Autodesk Inventor part; units mm, degrees
ref_plane "YZ Plane" through (0, 0, 0) normal (1, 0, 0) x (0, 1, 0)
ref_plane "XZ Plane" through (0, 0, 0) normal (0, 1, 0) x (-1, 0, 0)
ref_plane "XY Plane" through (0, 0, 0) normal (0, 0, 1) x (1, 0, 0)
sketch "Sketch1" plane through (0, 0, 0) normal (1, 0, 0) x (0, 1, 0)
  line L0 (-20, -30) -> (20, -30)
  line L1 (20, -30) -> (20, 30)
  line L2 (20, 30) -> (-20, 30)
  line L3 (-20, 30) -> (-20, -30)
  line L4 (-20, -30) -> (20, 30) construction
  line L5 (20, -30) -> (-20, 30) construction
  circle A0 centre (0, -30) radius 20
  point P0 (0, 0)
  dimension "d0" = 40
  dimension "d1" = 60
extrude "Extrusion1" add sketch "Sketch1" along normal blind 4
sketch "Sketch4" plane through (4, 0, 0) normal (1, 0, 0) x (0, 0, -1)
  line L0 (-5, 20) -> (-90, 20)
  line L1 (-90, 20) -> (-90, -50)
  line L2 (-90, -50) -> (-5, -50)
  line L3 (-5, -50) -> (-5, 20)
  line L4 (0, -64) -> (0, 34)
  line L5 (-10, -77.5279) -> (-10, 43.8166)
  dimension "d40" = 85
  dimension "d41" = 70
  dimension "d54" = 10
  dimension "d55" = 5
extrude "Extrusion4" add sketch "Sketch4" against normal blind 4
sketch "Sketch5" plane through (0, 0, 0) normal (-1, 0, 0) x (0, 0, 1)
  line L0 (34.5, -27) -> (24.2, -27)
  line L1 (24.2, -27) -> (24.2, -22.7)
  line L2 (24.2, -22.7) -> (34.5, -22.7)
  line L3 (34.5, -22.7) -> (34.5, -27)
  line L4 (90, -50) -> (90, -6.689)
  line L5 (90, -50) -> (90, 20)
  line L6 (90, -50) -> (10.2215, -50)
  line L7 (5, -50) -> (90, -50)
  dimension "d20" = 10.3
  dimension "d21" = 4.3
extrude "Extrusion5" cut sketch "Sketch5" against normal blind 4
sketch "Sketch2" plane through (0, 0, 0) normal (-1, 0, 0) x (0, 0, 1)
  arc A0 (-30, 20) -> (-30, -20) centre (-30, 0) ccw
  circle A1 centre (-30, 0) radius 5.15
  point P0 (0, 0)
  dimension "d4" = 10.3
extrude "Extrusion2" cut sketch "Sketch2" against normal blind 4
sketch "Sketch7" plane through (0, 0, 0) normal (-1, 0, 0) x (0, 0, 1)
  circle A0 centre (65, -7.5) radius 22.5
  line L0 (90, -50) -> (90, 20)
  line L1 (-30, 20) -> (90, 20)
  point P0 (0, 0)
  dimension "d47" = 45
  dimension "d48" = 25
  dimension "d53" = 27.5
extrude "Extrusion7" cut sketch "Sketch7" against normal blind 4
fillet "Fillet3" radius 15 2 edges at (2, -20, 5) (2, -50, 5)
properties part number "houder"
Read the model definition and answer for the solid it produces. Units are mm, in the model's axes. A direction names the side the tool comes from. Give positions to 0.01 mm unless a question says otherwise; leave off trailing zeros. Write each loop counter-clockwise with the first axis right and the second up, starting at its lowest first coordinate (ties: lowest second). Pieces come first, ordered by that corner, then holes. Notation, with made-up numbers: (84, 54.25) -> (107, 54.25) arc R21 cw to (107, 67.25) -> close; hole circle Ø4 at (89.25, 9.25). An arc over 180 degrees is marked (long way). Answer in a Markdown table with one row per item.
1) Section A-A on z = 65 is taken. Give the vertices of the cut face in (x, y), plus the area to 3 significant figures.
Results list:
| item | result |
|---|---|
| outline | (0, -50) -> (4, -50) -> (4, -30) -> (0, -30) -> close; (0, 15) -> (4, 15) -> (4, 20) -> (0, 20) -> close |
| area | 100 mm^2 |
2) Determine the mould class of faces 1 (the cylindrical face through (2, 0, -50)), 2 (the flat face through (4, -15, 21)), 3 (the flat face through (2, -25, 34.5)), 4 (the flat face through (2, -27, 29)) for opening direction Y: released by +Y, released by -Y, zero draft, split by the parting line, or undercut.
Results list:
| item | result |
|---|---|
| face 1 | split by the parting line |
| face 2 | zero draft |
| face 3 | undercut |
| face 4 | undercut |
3) Straight lines are drawn through the part: line 1 (Y direction, x = 2.25, z = -30); line 2 (Y direction, x = 2.1, z = 65); line 3 (Z direction, x = 3.15, y = -4). For each, find the intervals that lie inside material, in ascending order. Write a range as [from, to].
Results list:
| item | result |
|---|---|
| line 1 | [-20, -5.15], [5.15, 20] |
| line 2 | [-50, -30], [15, 20] |
| line 3 | [-49.6, -33.24], [-26.76, 42.77], [87.23, 90] |
4) Section C-C on y = -9 is taken. Give the vertices of the cut face in (x, z).
Results list:
| item | result |
|---|---|
| outline | (0, -47.86) -> (4, -47.86) -> (4, 42.55) -> (0, 42.55) -> close; (0, 87.45) -> (4, 87.45) -> (4, 90) -> (0, 90) -> close |
5) Section D-D on y = 0 is taken. Give the vertices of the cut face in (x, z).
Results list:
| item | result |
|---|---|
| outline | (0, -50) -> (4, -50) -> (4, -35.15) -> (0, -35.15) -> close; (0, -24.85) -> (4, -24.85) -> (4, 43.79) -> (0, 43.79) -> close; (0, 86.21) -> (4, 86.21) -> (4, 90) -> (0, 90) -> close |
6) A tool of negligible diameter and unlimited length cuts with its end or side. For faces 5 (the flat face through (2, -22.7, 29)), 6 (the flat face through (2, -20, -20)), 7 (the flat face through (2, 20, 29)), from which of +Z, -Z, +X, -X, +Y, -Y can it reach the whole face along a straight path? Write none if from no direction.
Results list:
| item | result |
|---|---|
| face 5 | +X, -X |
| face 6 | -Z, +X, -X, -Y |
| face 7 | +Z, -Z, +X, -X, +Y |
7) Section B-B on x = 0.6 is taken. Count the separate pieces of the cut face and the enclosed holes in it, plus the area to 3 significant figures.
Results list:
| item | result |
|---|---|
| separate pieces | 1 |
| enclosed holes | 3 |
| area | 6,260 mm^2 |
